```python
from build123d import *

# Parameters (mm, degrees)
F0_R     = 152.4
F1_DEPTH = 3.175


with BuildPart() as f1:
    # F0 (on Top) → F1 (new body)
    with BuildSketch(Plane.XY):
        Circle(F0_R)
        with BuildLine():
            ThreePointArc((-74.496722, -102.855425), (-77.10194, -98.215549), (-75.262014, -93.222526))
            Line((-75.262014, -93.222526), (-23.540128, -41.50064))
            ThreePointArc((-23.540128, -41.50064), (-16.61996, -40.124133), (-12.7, -45.990768))
            Line((-12.7, -45.990768), (-12.7, -119.13656))
            ThreePointArc((-12.7, -119.13656), (-14.929576, -123.968186), (-20.052632, -125.406906))
            ThreePointArc((-20.052632, -125.406906), (-48.600796, -117.332701), (-74.496722, -102.855425))
        make_face(mode=Mode.SUBTRACT)
        with BuildLine():
            ThreePointArc((-102.855425, -74.496722), (-117.332701, -48.600796), (-125.406906, -20.052632))
            ThreePointArc((-125.406906, -20.052632), (-123.968186, -14.929576), (-119.13656, -12.7))
            Line((-119.13656, -12.7), (-45.990768, -12.7))
            ThreePointArc((-45.990768, -12.7), (-40.124133, -16.61996), (-41.50064, -23.540128))
            Line((-41.50064, -23.540128), (-93.222526, -75.262014))
            ThreePointArc((-93.222526, -75.262014), (-98.215549, -77.10194), (-102.855425, -74.496722))
        make_face(mode=Mode.SUBTRACT)
        with BuildLine():
            ThreePointArc((20.052632, -125.406906), (14.929576, -123.968186), (12.7, -119.13656))
            Line((12.7, -119.13656), (12.7, -45.990768))
            ThreePointArc((12.7, -45.990768), (16.61996, -40.124133), (23.540128, -41.50064))
            Line((23.540128, -41.50064), (75.262014, -93.222526))
            ThreePointArc((75.262014, -93.222526), (77.10194, -98.215549), (74.496722, -102.855425))
            ThreePointArc((74.496722, -102.855425), (48.600796, -117.332701), (20.052632, -125.406906))
        make_face(mode=Mode.SUBTRACT)
        with BuildLine():
            ThreePointArc((119.13656, -12.7), (123.968186, -14.929576), (125.406906, -20.052632))
            ThreePointArc((125.406906, -20.052632), (117.332701, -48.600796), (102.855425, -74.496722))
            ThreePointArc((102.855425, -74.496722), (98.215549, -77.10194), (93.222526, -75.262014))
            Line((93.222526, -75.262014), (41.50064, -23.540128))
            ThreePointArc((41.50064, -23.540128), (40.124133, -16.61996), (45.990768, -12.7))
            Line((45.990768, -12.7), (119.13656, -12.7))
        make_face(mode=Mode.SUBTRACT)
        with BuildLine():
            Line((-45.990768, 12.7), (-119.13656, 12.7))
            ThreePointArc((-119.13656, 12.7), (-123.968186, 14.929576), (-125.406906, 20.052632))
            ThreePointArc((-125.406906, 20.052632), (-117.332701, 48.600796), (-102.855425, 74.496722))
            ThreePointArc((-102.855425, 74.496722), (-98.215549, 77.10194), (-93.222526, 75.262014))
            Line((-93.222526, 75.262014), (-41.50064, 23.540128))
            ThreePointArc((-41.50064, 23.540128), (-40.124133, 16.61996), (-45.990768, 12.7))
        make_face(mode=Mode.SUBTRACT)
        with BuildLine():
            ThreePointArc((-20.052632, 125.406906), (-14.929576, 123.968186), (-12.7, 119.13656))
            Line((-12.7, 119.13656), (-12.7, 45.990768))
            ThreePointArc((-12.7, 45.990768), (-16.61996, 40.124133), (-23.540128, 41.50064))
            Line((-23.540128, 41.50064), (-75.262014, 93.222526))
            ThreePointArc((-75.262014, 93.222526), (-77.10194, 98.215549), (-74.496722, 102.855425))
            ThreePointArc((-74.496722, 102.855425), (-48.600796, 117.332701), (-20.052632, 125.406906))
        make_face(mode=Mode.SUBTRACT)
        with BuildLine():
            ThreePointArc((102.855425, 74.496722), (117.332701, 48.600796), (125.406906, 20.052632))
            ThreePointArc((125.406906, 20.052632), (123.968186, 14.929576), (119.13656, 12.7))
            Line((119.13656, 12.7), (45.990768, 12.7))
            ThreePointArc((45.990768, 12.7), (40.124133, 16.61996), (41.50064, 23.540128))
            Line((41.50064, 23.540128), (93.222526, 75.262014))
            ThreePointArc((93.222526, 75.262014), (98.215549, 77.10194), (102.855425, 74.496722))
        make_face(mode=Mode.SUBTRACT)
        with BuildLine():
            ThreePointArc((74.496722, 102.855425), (77.10194, 98.215549), (75.262014, 93.222526))
            Line((75.262014, 93.222526), (23.540128, 41.50064))
            ThreePointArc((23.540128, 41.50064), (16.61996, 40.124133), (12.7, 45.990768))
            Line((12.7, 45.990768), (12.7, 119.13656))
            ThreePointArc((12.7, 119.13656), (14.929576, 123.968186), (20.052632, 125.406906))
            ThreePointArc((20.052632, 125.406906), (48.600796, 117.332701), (74.496722, 102.855425))
        make_face(mode=Mode.SUBTRACT)
    extrude(amount=F1_DEPTH)


solid = f1.part
```
For this review, take the finished solid that the model builds, in its own axes (mm). A direction names the side the tool comes from. Give positions to 0.01 mm unless a question says otherwise; leave off trailing zeros. Write each loop counter-clockwise with the first axis right and the second up, starting at its lowest first coordinate (ties: lowest second). Pieces come first, ordered by that corner, then holes.
Item 1: Take a section at C-C (z = 1.7). Give the number of separate pieces and of enclosed holes in the cut face, and give its area (3 significant figures).
Item 2: Insertion check: P1, Ø1.6, axis at y = 69, z = 1, coming from the +X side; P2, Ø3, axis at x = 75, y = -57.5, coming from the -Z side; P3, Ø1.6, axis at y = -84, z = 1.5, coming from the +X side; P4, Ø1.6, axis at x = -99.5, z = 1.5, coming from the -Y side. Each pin has a flat end and moves straight along its axis. Give the tip position at first contact, or say it passes through.
Item 3: Wall thickness on probe 1 along Y at (x, z) = (-83.5, 2.3); probe 2 along Y at (x, z) = (24.5, 2.3); probe 3 along Y at (x, z) = (48, 2): over which ranges is each line inside the solid? List them lowest first.
Item 4: Take a section at B-B (y = -88.5). Give the boundary of the cut face in (x, z) (3 decimals), and give its area (3 significant figures).
Item 5: Machinability: for faces 1 (the face through (67, 49.04, 1.57)), 2 (the face through (-2, 2, 3.175)), which of the approach directions +Z, -Z, +X, -X, +Y, -Y give a long, thin tool a straight path to every point of the face, cutting with its end or side? Answer none if there is none.
Item 6: Take a section at A-A (x = 28). Give the boundary of the cut face in (y, z) (3 decimals), and give its area (3 significant figures).
Item 7: The part is to be moulded in two halves that separate along Y. For faces 3 (the face through (-2, 2, 0)), 4 (the face through (-49.04, 67, 1.57)), 5 (the face through (67.72, -49.76, 1.57)), 6 (the face through (-120.94, -92.73, 1.57)), say which applies: +Y half, -Y half, draft (parallel to the pull), parting line (faces both ways), or undercut.
Established:
1. separate pieces: 1
1. enclosed holes: 8
1. area: 45,500 mm2
2. P1: stops at x = 136.29
2. P2: stops at z = 0
2. P3: stops at x = 127.69
2. P4: stops at y = -116.12
3. probe 1: y = -127.49 to -65.54, -12.7 to 12.7, 65.54 to 127.49
3. probe 2: y = -150.42 to -124.61, -42.46 to 42.46, 124.61 to 150.42
3. probe 3: y = -144.64 to -117.58, -65.96 to -30.04, -12.7 to 12.7, 30.04 to 65.96, 117.58 to 144.64
4. outline: (-124.071, 0) - (-70.539, 0) - (-70.539, 3.175) - (-124.071, 3.175) - close; (-12.7, 0) - (12.7, 0) - (12.7, 3.175) - (-12.7, 3.175) - close; (70.539, 0) - (124.071, 0) - (124.071, 3.175) - (70.539, 3.175) - close
4. area: 421 mm2
5. face 1: +Z, -Z
5. face 2: +Z, +X, -X, +Y, -Y
6. outline: (-149.806, 0) - (-123.875, 0) - (-123.875, 3.175) - (-149.806, 3.175) - close; (-45.961, 0) - (45.961, 0) - (45.961, 3.175) - (-45.961, 3.175) - close; (123.875, 0) - (149.806, 0) - (149.806, 3.175) - (123.875, 3.175) - close
6. area: 457 mm2
7. face 3: draft
7. face 4: undercut
7. face 5: undercut
7. face 6: parting line
